Autodesk Inventor part; units mm, degrees
ref_plane "YZ Plane" through (0, 0, 0) normal (1, 0, 0) x (0, 1, 0)
ref_plane "XZ Plane" through (0, 0, 0) normal (0, 1, 0) x (-1, 0, 0)
ref_plane "XY Plane" through (0, 0, 0) normal (0, 0, 1) x (1, 0, 0)
sketch "Sketch1" plane through (0, 0, 0) normal (0, 1, 0) x (-1, 0, 0)
  line L0 (0, -4.739) -> (0, 4.739) construction
  line L1 (4.2, 0) -> (-4.2, 0) construction
  line L2 (3, 1.7164) -> (3, -1.7164)
  line L3 (3, -1.7164) -> (0, -3.385)
  line L4 (0, -3.385) -> (-3, -1.7164)
  line L5 (-3, -1.7164) -> (-3, 1.7164)
  line L6 (-3, 1.7164) -> (0, 3.385)
  line L7 (0, 3.385) -> (3, 1.7164)
  point P0 (3, 0)
  point P1 (-3, 0)
  dimension "d2" = 6.77
  dimension "d3" = 6
extrude "Extrusion1" add sketch "Sketch1" along normal blind 13
fillet "Fillet1" radius 0.5 6 edges at (0, 6.5, 3.385) (3, 6.5, 1.7164) (3, 6.5, -1.7164) (0, 6.5, -3.385) (-3, 6.5, -1.7164) (-3, 6.5, 1.7164)
sketch "Sketch2" plane through (0, 0, 0) normal (0, 0, 1) x (1, 0, 0)
  line L0 (-0.243, 13) -> (0.243, 13)
  line L1 (0, 13) -> (-0.1, 13)
  line L2 (-0.1, 13) -> (-0.6, 13)
  line L3 (-0.6, 13) -> (-3, 9.0992)
  line L4 (-0.243, 13) -> (-2.743, 13)
  line L5 (0, 13) -> (0, 13.665)
  line L6 (-0.6, 13) -> (-4.1, 13)
  line L7 (-4.1, 13) -> (-4.1, 7.3113)
  line L8 (-3, 13) -> (-3, 0)
  line L9 (-4.1, 7.3113) -> (-3, 9.0992)
  point P0 (0, 0)
  dimension "d7" = 0.1
  dimension "d8" = 0.5
  dimension "d9" = 4.58
  dimension "d11" = 3.5
revolve "Revolution1" cut sketch "Sketch2" angle 360 about axis through (0, 13, 0) along (0, 1, 0)
sketch "Sketch3" plane through (0, 0, 0) normal (0, -1, 0) x (1, 0, 0)
  circle A0 centre (0, 0) radius 2.5
  arc A1 (-2.743, 1.8593) -> (-3, 1.4224) centre (-2.5, 1.4224) ccw
  line L0 (-3, -1.4224) -> (-3, 1.4224)
  arc A2 (-3, -1.4224) -> (-2.743, -1.8593) centre (-2.5, -1.4224) ccw
  line L1 (-0.243, -3.2498) -> (-2.743, -1.8593)
  arc A3 (-0.243, -3.2498) -> (0.243, -3.2498) centre (0, -2.8129) ccw
  line L2 (2.743, -1.8593) -> (0.243, -3.2498)
  arc A4 (2.743, -1.8593) -> (3, -1.4224) centre (2.5, -1.4224) ccw
  line L3 (3, 1.4224) -> (3, -1.4224)
  arc A5 (3, 1.4224) -> (2.743, 1.8593) centre (2.5, 1.4224) ccw
  line L4 (0.243, 3.2498) -> (2.743, 1.8593)
  arc A6 (0.243, 3.2498) -> (-0.243, 3.2498) centre (0, 2.8129) ccw
  line L5 (-2.743, 1.8593) -> (-0.243, 3.2498)
  dimension "d12" = 5
extrude "Extrusion2" cut sketch "Sketch3" against normal blind 5
thread "Thread1"
sketch "Sketch4" plane through (0, 0, 0) normal (0, -1, 0) x (1, 0, 0)
  circle A0 centre (0, 0) radius 0.6
  circle A1 centre (0, 0) radius 1
  point P0 (0, 0)
  dimension "d20" = 2
extrude "Extrusion3" cut sketch "Sketch4" against normal blind 11 contours A0 | A1
sketch "Sketch5" plane through (0, 0, 0) normal (0, 0, 1) x (1, 0, 0)
  line L0 (1, 11) -> (-1, 11)
  line L1 (-1, 11) -> (-0.2, 12.51)
  line L2 (1, 11) -> (0.2, 12.51)
  line L3 (-0.2, 12.51) -> (0.2, 12.51) construction
  line L4 (0, -2.6) -> (0, 15.6)
  line L5 (0.6, 13) -> (-0.6, 13)
  line L6 (0.2, 12.51) -> (0.2, 13.1094)
  line L7 (0.2, 13.1094) -> (-0.2, 13.1094)
  line L8 (-0.2, 13.1094) -> (-0.2, 12.51)
  point P0 (0, 0)
  point P1 (0, 12.51)
  point P2 (0, 13.1094)
  point P3 (0, 11)
  dimension "d25" = 0.4
  dimension "d26" = 1.51
revolve "Revolution2" cut sketch "Sketch5" angle 360 about axis through (0, -10, 0) along (0, 1, 0) contours L0 L4 L5 L6 L2 | L4 L7 L6 L5
properties part number "Nozzle 0.4mm" material "Brass, Soft Yellow"
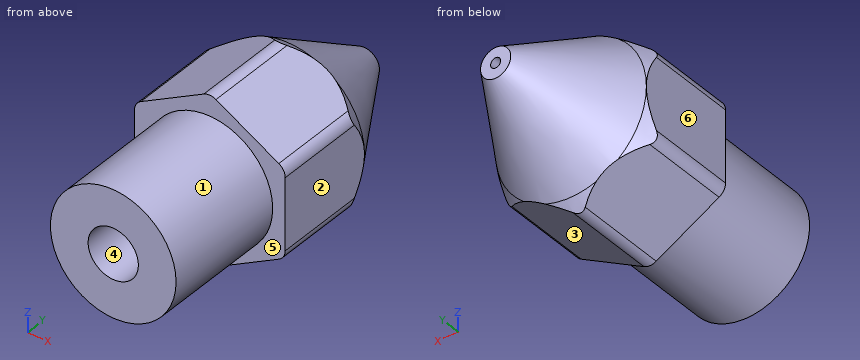
Work out the finished part from the listing and answer in its coordinate system (mm). Face numbers are marked on the shaded views. A direction names the side the tool comes from. Coordinates: 2 decimals unless noted, no trailing zeros. Loops run counter-clockwise (first coordinate to the right, second up) from the corner with the lowest first, then second, coordinate; pieces in that order, holes last. Notation, with made-up numbers: (41.5, 36.25) - (54.5, 36.25) arc R17 ccw to (54.5, 48.25) - close; hole circle Ø9 at (82.25, 65). An arc over 180 degrees is marked (long way). Use a Markdown table: item, result.
Item 1: Find section A-A, the plane x = 0. Determine the outline of the cut face in (y, z).
Evaluation:
| item | result |
|---|---|
| outline | (0, -2.5) - (5, -2.5) - (5, -3.31) - (8.59, -3.31) - (9.1, -3) - (13, -0.6) - (13, -0.2) - (12.51, -0.2) - (11, -1) - (0, -1) - close; (0, 1) - (11, 1) - (12.51, 0.2) - (13, 0.2) - (13, 0.6) - (9.1, 3) - (8.59, 3.31) - (5, 3.31) - (5, 2.5) - (0, 2.5) - close |
Item 2: Consider probe 1 along Z at (x, y) = (0, 5.75); probe 2 along X at (y, z) = (2, -0.5); probe 3 along Z at (x, y) = (0, 12.7). Determine where each line is inside the solid, lowest interval first. Write a range as from..to.
Evaluation:
| item | result |
|---|---|
| probe 1 | z = -3.31..-1, 1..3.31 |
| probe 2 | x = -2.45..-0.87, 0.87..2.45 |
| probe 3 | z = -0.78..-0.2, 0.2..0.78 |
Item 3: Find section B-B, the plane y = 7.25. Determine the outline of the cut face in (x, z).
Evaluation:
| item | result |
|---|---|
| outline | (-3, -1.42) arc R0.5 ccw to (-2.74, -1.86) - (-0.24, -3.25) arc R0.5 ccw to (0.24, -3.25) - (2.74, -1.86) arc R0.5 ccw to (3, -1.42) - (3, 1.42) arc R0.5 ccw to (2.74, 1.86) - (0.24, 3.25) arc R0.5 ccw to (-0.24, 3.25) - (-2.74, 1.86) arc R0.5 ccw to (-3, 1.42) - close; hole circle Ø2 at (0, 0) |
Item 4: The mould has two halves that part along Z. Classify the marked faces 1, 2, 3 and 4: +Z half, -Z half, draft (parallel to the pull), parting line (faces both ways), or undercut.
Evaluation:
| item | result |
|---|---|
| face 1 | parting line |
| face 2 | draft |
| face 3 | -Z half |
| face 4 | undercut |
Item 5: Find section C-C, the plane y = 3.25. Determine the outline of the cut face in (x, z), and give its area (3 significant figures).
Evaluation:
| item | result |
|---|---|
| outline | circle Ø5 at (0, 0); hole circle Ø2 at (0, 0) |
| area | 16.5 mm2 |
Item 6: For the marked faces 5 and 6, determine the directions among +Z, -Z, +X, -X, +Y, -Y from which every point of the face is accessible in a straight line to the end or side of a thin tool.
Evaluation:
| item | result |
|---|---|
| face 5 | -Y |
| face 6 | +Z, -Z, -X, +Y, -Y |
